Part model, mm, in its own coordinate system. Coordinates: 2 decimals unless noted, no trailing zeros. Order: outer loops, then holes, each group sorted by start corner. A loop starts at its lowest first (then second) coordinate and runs counter-clockwise, first axis right, second up.
1) Cut at B-B (x = 77). List the corners of the cut face in (y, z) (3 decimals), and give its area (3 significant figures).
2) Cut at A-A (y = 55.5). List the corners of the cut face in (x, z) (1 decimal), and give its area (3 significant figures).
3) Cut at C-C (y = -112). List the corners of the cut face in (x, z) (1 decimal).
4) Cut at D-D (z = 0.6). Give the number of separate pieces and of enclosed holes in the cut face, and give its area (3 significant figures).
5) Wall check: L1, parallel to X at y = -89, z = 0.3; L2, parallel to X at y = -154, z = 0.6; L3, parallel to X at y = -60, z = 2.4. Give the ranges that are in metal, low to high.
6) Pin check, flat tips, straight feed: pin 1 Ø1.6 at (x, z) = (-261.5, 1.5) entering from -Y; pin 2 Ø1.6 at (y, z) = (-204.5, 2) entering from +X; pin 3 Ø6.5 at (x, y) = (-254.01, -135.59) entering from +Z. Stop position of each tip, or through.
```python
from build123d import *

# Parameters (mm, degrees)
SKETCH1_W            = 457.223
SKETCH1_H            = 367.60800004
BOSS_EXTRUDE2_DEPTH  = 3.175
SKETCH8_W            = 44.275
SKETCH8_H            = 95.25
SKETCH8_W_2          = 93.98
SKETCH8_H_2          = 44.45
BOSS_EXTRUDE3_DEPTH  = 3.175
M6_CLEARANCE_HOLE1_D = 7
SKETCH12_W           = 3.184
SKETCH12_H           = 57.15
SKETCH12_W_2         = 3.175
SKETCH12_H_2         = 26.9875
SKETCH12_W_3         = 50.9524
SKETCH12_H_3         = 3.3274
SKETCH12_W_4         = 50.8
SKETCH12_H_4         = 3.175
SKETCH12_W_5         = 3.179
CUT_EXTRUDE3_DEPTH   = 345.589489363
SKETCH14_W           = 3.3274
SKETCH14_H           = 101.7524
SKETCH14_W_2         = 3.175
SKETCH14_H_2         = 101.6
CUT_EXTRUDE4_DEPTH   = 345.589489363
LPATTERN2_COUNT      = 4
LPATTERN2_PITCH      = 90.806999996
SKETCH16_W           = 9.6774
SKETCH16_H           = 6.5024
SKETCH16_W_2         = 9.525
SKETCH16_H_2         = 6.35
CUT_EXTRUDE5_DEPTH   = 345.589489363


with BuildPart() as part:
    # Sketch1 → Boss-Extrude2 (new body)
    with BuildSketch(Plane.XY):
        with Locations((0, -26.588)):
            Rectangle(SKETCH1_W, SKETCH1_H)
    extrude(amount=BOSS_EXTRUDE2_DEPTH)

    # Sketch8 → Boss-Extrude3 (add)
    with BuildSketch(Plane(origin=(0, 0, 0), x_dir=(-1, 0, 0), z_dir=(0, 0, -1))):
        with Locations((-250.749, 109.59100002)):
            Rectangle(SKETCH8_W, SKETCH8_H)
        with Locations((-181.6215, 179.44100002)):
            Rectangle(SKETCH8_W_2, SKETCH8_H_2)
        with Locations((-250.749, -109.59100002)):
            Rectangle(SKETCH8_W, SKETCH8_H)
    boss_extrude3 = extrude(amount=-BOSS_EXTRUDE3_DEPTH)

    # Mirror7: Boss-Extrude3 across plane
    add(boss_extrude3.mirror(Plane(origin=(0, 0, 0), x_dir=(0, 0, 1), z_dir=(1, 0, 0))))

    # M6 Clearance Hole1 (through all)
    with Locations(Plane(origin=(0, 0, 0), x_dir=(-1, 0, 0), z_dir=(0, 0, -1))):
        with Locations((-254.0115, -135.59100002), (-254.0115, -83.59100002), (-254.0115, 83.59100002), (-254.0115, 135.59100002), (-181.6215, 179.44100002)):
            m6_clearance_hole1 = Hole(M6_CLEARANCE_HOLE1_D / 2)

    # Mirror8: M6 Clearance Hole1 across plane
    add(m6_clearance_hole1.mirror(Plane(origin=(0, 0, 0), x_dir=(0, 0, 1), z_dir=(1, 0, 0))), mode=Mode.SUBTRACT)

    # Sketch12 → Cut-Extrude3 (cut, through all)
    # profile 1 of 16: a face of its own
    with BuildSketch(Plane(origin=(0, 0, 0), x_dir=(-1, 0, 0), z_dir=(0, 0, -1))):
        with Locations((-227.0195, 0)):
            Rectangle(SKETCH12_W, SKETCH12_H)
    # profile 2 of 16: a face of its own
    with BuildSketch(Plane(origin=(0, 0, 0), x_dir=(-1, 0, 0), z_dir=(0, 0, -1))):
        Polygon((-228.6115, 28.6512), (-228.6115, 28.575), (-225.4275, 28.575), (-225.4275, -28.575), (-228.6115, -28.575), (-228.6115, -28.6512), (-225.3513, -28.6512), (-225.3513, 28.6512), align=None)
    # profile 3 of 16: a face of its own
    with BuildSketch(Plane(origin=(0, 0, 0), x_dir=(-1, 0, 0), z_dir=(0, 0, -1))):
        with Locations((-227.024, -182.66100002)):
            Rectangle(SKETCH12_W_2, SKETCH12_H_2)
    # profile 4 of 16: a face of its own
    with BuildSketch(Plane(origin=(0, 0, 0), x_dir=(-1, 0, 0), z_dir=(0, 0, -1))):
        Polygon((-228.6115, -196.15475002), (-228.6115, -196.23095002), (-225.3603, -196.23095002), (-225.3603, -169.09105002), (-228.6115, -169.09105002), (-228.6115, -169.16725002), (-225.4365, -169.16725002), (-225.4365, -196.15475002), align=None)
    # profile 5 of 16: a face of its own
    with BuildSketch(Plane(origin=(0, 0, 0), x_dir=(-1, 0, 0), z_dir=(0, 0, -1))):
        with Locations((-90.8045, -155.62850002)):
            Rectangle(SKETCH12_W_3, SKETCH12_H_3)
        with Locations((-90.8045, -155.62850002)):
            Rectangle(SKETCH12_W_4, SKETCH12_H_4, mode=Mode.SUBTRACT)
    # profile 6 of 16: a face of its own
    with BuildSketch(Plane(origin=(0, 0, 0), x_dir=(-1, 0, 0), z_dir=(0, 0, -1))):
        with Locations((-90.8045, -155.62850002)):
            Rectangle(SKETCH12_W_4, SKETCH12_H_4)
    # profile 7 of 16: a face of its own
    with BuildSketch(Plane(origin=(0, 0, 0), x_dir=(-1, 0, 0), z_dir=(0, 0, -1))):
        with Locations((90.8095, -155.62850002)):
            Rectangle(SKETCH12_W_3, SKETCH12_H_3)
        with Locations((90.8095, -155.62850002)):
            Rectangle(SKETCH12_W_4, SKETCH12_H_4, mode=Mode.SUBTRACT)
    # profile 8 of 16: a face of its own
    with BuildSketch(Plane(origin=(0, 0, 0), x_dir=(-1, 0, 0), z_dir=(0, 0, -1))):
        with Locations((90.8095, -155.62850002)):
            Rectangle(SKETCH12_W_4, SKETCH12_H_4)
    # profile 9 of 16: a face of its own
    with BuildSketch(Plane(origin=(0, 0, 0), x_dir=(-1, 0, 0), z_dir=(0, 0, -1))):
        with Locations((227.024, -182.66100002)):
            Rectangle(SKETCH12_W_2, SKETCH12_H_2)
    # profile 10 of 16: a face of its own
    with BuildSketch(Plane(origin=(0, 0, 0), x_dir=(-1, 0, 0), z_dir=(0, 0, -1))):
        Polygon((225.3603, -196.23095002), (228.6115, -196.23095002), (228.6115, -196.15475002), (225.4365, -196.15475002), (225.4365, -169.16725002), (228.6115, -169.16725002), (228.6115, -169.09105002), (225.3603, -169.09105002), align=None)
    # profile 11 of 16: a face of its own
    with BuildSketch(Plane(origin=(0, 0, 0), x_dir=(-1, 0, 0), z_dir=(0, 0, -1))):
        with Locations((227.022, 0)):
            Rectangle(SKETCH12_W_5, SKETCH12_H)
    # profile 12 of 16: a face of its own
    with BuildSketch(Plane(origin=(0, 0, 0), x_dir=(-1, 0, 0), z_dir=(0, 0, -1))):
        Polygon((225.4325, -28.575), (225.4325, 28.575), (228.6115, 28.575), (228.6115, 28.6512), (225.3563, 28.6512), (225.3563, -28.6512), (228.6115, -28.6512), (228.6115, -28.575), align=None)
    # profile 13 of 16: a face of its own
    with BuildSketch(Plane(origin=(0, 0, 0), x_dir=(-1, 0, 0), z_dir=(0, 0, -1))):
        with Locations((90.8095, 155.62850002)):
            Rectangle(SKETCH12_W_4, SKETCH12_H_4)
    # profile 14 of 16: a face of its own
    with BuildSketch(Plane(origin=(0, 0, 0), x_dir=(-1, 0, 0), z_dir=(0, 0, -1))):
        Polygon((65.4095, 157.21600002), (65.3333, 157.21600002), (65.3333, 153.96480002), (116.2857, 153.96480002), (116.2857, 157.21600002), (116.2095, 157.21600002), (116.2095, 154.04100002), (65.4095, 154.04100002), align=None)
    # profile 15 of 16: a face of its own
    with BuildSketch(Plane(origin=(0, 0, 0), x_dir=(-1, 0, 0), z_dir=(0, 0, -1))):
        with Locations((-90.8045, 155.62850002)):
            Rectangle(SKETCH12_W_4, SKETCH12_H_4)
    # profile 16 of 16: a face of its own
    with BuildSketch(Plane(origin=(0, 0, 0), x_dir=(-1, 0, 0), z_dir=(0, 0, -1))):
        Polygon((-116.2045, 154.04100002), (-116.2045, 157.21600002), (-116.2807, 157.21600002), (-116.2807, 153.96480002), (-65.3283, 153.96480002), (-65.3283, 157.21600002), (-65.4045, 157.21600002), (-65.4045, 154.04100002), align=None)
    extrude(amount=-CUT_EXTRUDE3_DEPTH, mode=Mode.SUBTRACT)

    # Sketch14 → Cut-Extrude4 (cut, through all)
    # profile 1 of 4: a face of its own
    with BuildSketch(Plane(origin=(0, 0, 0), x_dir=(-1, 0, 0), z_dir=(0, 0, -1))):
        with Locations((-136.208, 77.02050001)):
            Rectangle(SKETCH14_W, SKETCH14_H)
        with Locations((-136.208, 77.02050001)):
            Rectangle(SKETCH14_W_2, SKETCH14_H_2, mode=Mode.SUBTRACT)
    # profile 2 of 4: a face of its own
    with BuildSketch(Plane(origin=(0, 0, 0), x_dir=(-1, 0, 0), z_dir=(0, 0, -1))):
        with Locations((-136.208, 77.02050001)):
            Rectangle(SKETCH14_W_2, SKETCH14_H_2)
    # profile 3 of 4: a face of its own
    with BuildSketch(Plane(origin=(0, 0, 0), x_dir=(-1, 0, 0), z_dir=(0, 0, -1))):
        with Locations((-136.208, -77.02050001)):
            Rectangle(SKETCH14_W, SKETCH14_H)
        with Locations((-136.208, -77.02050001)):
            Rectangle(SKETCH14_W_2, SKETCH14_H_2, mode=Mode.SUBTRACT)
    # profile 4 of 4: a face of its own
    with BuildSketch(Plane(origin=(0, 0, 0), x_dir=(-1, 0, 0), z_dir=(0, 0, -1))):
        with Locations((-136.208, -77.02050001)):
            Rectangle(SKETCH14_W_2, SKETCH14_H_2)
    cut_extrude4 = extrude(amount=-CUT_EXTRUDE4_DEPTH, mode=Mode.SUBTRACT)

    # LPattern2: Cut-Extrude4 ×4
    with Locations(*[(-i * LPATTERN2_PITCH, 0, 0) for i in range(1, LPATTERN2_COUNT)]):
        add(cut_extrude4, mode=Mode.SUBTRACT)

    # Sketch16 → Cut-Extrude5 (cut, through all)
    # profile 1 of 6: a face of its own
    with BuildSketch(Plane.XY.offset(3.175)):
        with Locations((152.4, -204.92974)):
            Rectangle(SKETCH16_W, SKETCH16_H)
        with Locations((152.4, -204.92974)):
            Rectangle(SKETCH16_W_2, SKETCH16_H_2, mode=Mode.SUBTRACT)
    # profile 2 of 6: a face of its own
    with BuildSketch(Plane.XY.offset(3.175)):
        with Locations((152.4, -204.92974)):
            Rectangle(SKETCH16_W_2, SKETCH16_H_2)
    # profile 3 of 6: a face of its own
    with BuildSketch(Plane.XY.offset(3.175)):
        with Locations((0, -204.92974)):
            Rectangle(SKETCH16_W, SKETCH16_H)
        with Locations((0, -204.92974)):
            Rectangle(SKETCH16_W_2, SKETCH16_H_2, mode=Mode.SUBTRACT)
    # profile 4 of 6: a face of its own
    with BuildSketch(Plane.XY.offset(3.175)):
        with Locations((0, -204.92974)):
            Rectangle(SKETCH16_W_2, SKETCH16_H_2)
    # profile 5 of 6: a face of its own
    with BuildSketch(Plane.XY.offset(3.175)):
        with Locations((-152.4, -204.92974)):
            Rectangle(SKETCH16_W, SKETCH16_H)
        with Locations((-152.4, -204.92974)):
            Rectangle(SKETCH16_W_2, SKETCH16_H_2, mode=Mode.SUBTRACT)
    # profile 6 of 6: a face of its own
    with BuildSketch(Plane.XY.offset(3.175)):
        with Locations((-152.4, -204.92974)):
            Rectangle(SKETCH16_W_2, SKETCH16_H_2)
    extrude(amount=-CUT_EXTRUDE5_DEPTH, mode=Mode.SUBTRACT)


solid = part.part
```
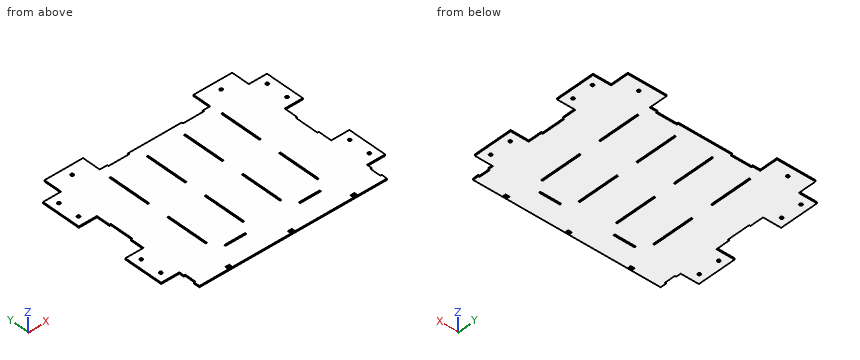
Geometry check:
1. outline: (-210.392, 0) - (-157.292, 0) - (-157.292, 3.175) - (-210.392, 3.175) - close; (-153.965, 0) - (153.965, 0) - (153.965, 3.175) - (-153.965, 3.175) - close
1. area: 1,150 mm2
2. outline: (-228.6, 0) - (-137.9, 0) - (-137.9, 3.2) - (-228.6, 3.2) - close; (-134.5, 0) - (-47.1, 0) - (-47.1, 3.2) - (-134.5, 3.2) - close; (-43.7, 0) - (43.7, 0) - (43.7, 3.2) - (-43.7, 3.2) - close; (47.1, 0) - (134.5, 0) - (134.5, 3.2) - (47.1, 3.2) - close; (137.9, 0) - (228.6, 0) - (228.6, 3.2) - (137.9, 3.2) - close
2. area: 1,410 mm2
3. outline: (-272.9, 0) - (-137.9, 0) - (-137.9, 3.2) - (-272.9, 3.2) - close; (-134.5, 0) - (-47.1, 0) - (-47.1, 3.2) - (-134.5, 3.2) - close; (-43.7, 0) - (43.7, 0) - (43.7, 3.2) - (-43.7, 3.2) - close; (47.1, 0) - (134.5, 0) - (134.5, 3.2) - (47.1, 3.2) - close; (137.9, 0) - (272.9, 0) - (272.9, 3.2) - (137.9, 3.2) - close
4. separate pieces: 1
4. enclosed holes: 23
4. area: 189,000 mm2
5. L1: x = -272.89 to -137.88, -134.55 to -47.07, -43.74 to 43.74, 47.06 to 134.54, 137.87 to 272.89
5. L2: x = -272.89 to -116.29, -65.33 to 65.33, 116.28 to 272.89
5. L3: x = -228.61 to -137.88, -134.55 to -47.07, -43.74 to 43.74, 47.06 to 134.54, 137.87 to 228.61
6. pin 1: stops at y = -157.22
6. pin 2: stops at x = 228.61
6. pin 3: passes through
